```python
from build123d import *

# Parameters (mm, degrees)
F0_W      = 25.4
F0_H      = 25.4
F1_DEPTH  = 25.4
F2_W      = 20.32
F2_H      = 22.86
F3_DEPTH  = 7.62
F4_W      = 3.556
F4_H      = 20.32
F5_DEPTH  = 3.048
F6_W      = 3.556
F6_H      = 19.812
F7_DEPTH  = 3.048
F8_W      = 3.556
F8_H      = 19.812
F9_DEPTH  = 3.048
F13_DEPTH = 23.368
F12_W     = 2.54
F12_H     = 15.24
F14_DEPTH = 20.32


with BuildPart() as f1:
    # F0 (on Top) → F1 (new body)
    with BuildSketch(Plane.XY):
        Rectangle(F0_W, F0_H)
    extrude(amount=F1_DEPTH)

    # F2 (on face) → F3 (join)
    with BuildSketch(Plane(origin=(-12.7, 0, 0), x_dir=(0, -1, 0), z_dir=(-1, 0, 0))):
        with Locations((0, 11.43)):
            Rectangle(F2_W, F2_H)
    extrude(amount=F3_DEPTH)

    # F4 (on face) → F5 (cut)
    with BuildSketch(Plane.XY.offset(22.86)):
        with Locations((-16.51, 0)):
            Rectangle(F4_W, F4_H)
    extrude(amount=-F5_DEPTH, mode=Mode.SUBTRACT)

    # F6 (on face) → F7 (cut)
    with BuildSketch(Plane.XZ.offset(10.16)):
        with Locations((-16.51, 9.906)):
            Rectangle(F6_W, F6_H)
    extrude(amount=-F7_DEPTH, mode=Mode.SUBTRACT)

    # F8 (on face) → F9 (cut)
    with BuildSketch(Plane(origin=(0, 10.16, 0), x_dir=(-1, 0, 0), z_dir=(0, 1, 0))):
        with Locations((16.51, 9.906)):
            Rectangle(F8_W, F8_H)
    extrude(amount=-F9_DEPTH, mode=Mode.SUBTRACT)

    # F12 (on face) → F13 (cut)
    with BuildSketch(Plane(origin=(0, 0, 0), x_dir=(1, 0, 0), z_dir=(0, 0, -1))):
        Polygon((10.16, -7.62), (10.16, 7.62), (10.16, 10.668), (7.62, 10.668), (7.62, -10.668), (10.16, -10.668), align=None)
    extrude(amount=-F13_DEPTH, mode=Mode.SUBTRACT)

    # F12 (on face) → F14 (cut)
    with BuildSketch(Plane(origin=(0, 0, 0), x_dir=(1, 0, 0), z_dir=(0, 0, -1))):
        with Locations((11.43, 0)):
            Rectangle(F12_W, F12_H)
    extrude(amount=-F14_DEPTH, mode=Mode.SUBTRACT)


with BuildPart() as f10_1:
    # F10: copy of F1
    add(f1.part.moved(Location((-54.102, 0, 0))))


solid = f1.part
```
Model file for the job. Use its own axes, mm. A direction names the side the tool comes from. Coordinates: 2 decimals unless noted, no trailing zeros. Order: outer loops, then holes, each group sorted by start corner. A loop starts at its lowest first (then second) coordinate and runs counter-clockwise, first axis right, second up. Notation, with made-up numbers: (-19, -32.5) - (21, -32.5) arc R8 cw to (21, -24.5) - close; hole circle Ø4 at (15, -32.5). An arc over 180 degrees is marked (long way). Return JSON: item names as keys, results as strings. Group by question number.
1) Probe line 1 (X direction, y = -3.5, z = 21); line 2 (X direction, y = -7.25, z = 2); line 3 (Y direction, x = 11, z = 9.5). List the from-to ranges inside material, lowest first. Write a range as from..to.
2) Saw through at B-B, the plane z = 21.5. Write the cut outline in (x, y).
3) Mould opens along X. For faces 4 (the flat face through (-20.32, 0, 12)), 5 (the flat face through (11, 7.62, 10)), 6 (the flat face through (-17, -7.112, 10)) say: released by +X, released by -X, zero draft, split by the parting line, or undercut.
4) Tool access for faces 1 (the flat face through (9, 10.668, 12)), 2 (the flat face through (-14, -10.16, 11)), 3 (the flat face through (11, 0, 20.32)): list every direction of +Z, -Z, +X, -X, +Y, -Y with a clear straight run to the whole face (end or side of a thin tool).
5) Saw through at C-C, the plane y = -1.25. Write the cut outline in (x, z), plus the area to 3 significant figures.
6) Saw through at D-D, the plane z = 8.75. Write the cut outline in (x, y).
7) Saw through at A-A, the plane y = 9.5. Write the cut outline in (x, z), plus the area to 3 significant figures.
8) Flat gauge pins, fed straight in: P1, Ø1, axis at x = -14, z = 6.5, coming from the -Y side; P2, Ø5, axis at y = 3.5, z = 11.5, coming from the +X side; P3, Ø1.5, axis at x = -14.5, z = 17.5, coming from the +Y side. Where does each tip first touch, or does it go through?
Values found:
{
 "1": {"line 1": "x = -20.32..-18.29, -14.73..7.62, 10.16..12.7", "line 2": "x = -20.32..-18.29, -14.73..7.62", "line 3": "y = -12.7..-7.62, 7.62..12.7"},
 "2": {"outline": "(-20.32, -10.16) - (-18.29, -10.16) - (-18.29, 10.16) - (-20.32, 10.16) - close; (-14.73, -10.16) - (-12.7, -10.16) - (-12.7, -12.7) - (12.7, -12.7) - (12.7, 12.7) - (-12.7, 12.7) - (-12.7, 10.16) - (-14.73, 10.16) - close; hole (7.62, -10.67) - (10.16, -10.67) - (10.16, 10.67) - (7.62, 10.67) - close"},
 "3": {"face 4": "released by -X", "face 5": "zero draft", "face 6": "undercut"},
 "4": {"face 1": "-Z", "face 2": "+Z, -Z, -X, -Y", "face 3": "-Z, +X"},
 "5": {"outline": "(-20.32, 0) - (7.62, 0) - (7.62, 23.37) - (10.16, 23.37) - (10.16, 20.32) - (12.7, 20.32) - (12.7, 25.4) - (-12.7, 25.4) - (-12.7, 22.86) - (-14.73, 22.86) - (-14.73, 19.81) - (-18.29, 19.81) - (-18.29, 22.86) - (-20.32, 22.86) - close", "area": "698 mm²"},
 "6": {"outline": "(-20.32, -10.16) - (-18.29, -10.16) - (-18.29, -7.11) - (-14.73, -7.11) - (-14.73, -10.16) - (-12.7, -10.16) - (-12.7, -12.7) - (12.7, -12.7) - (12.7, -7.62) - (10.16, -7.62) - (10.16, -10.67) - (7.62, -10.67) - (7.62, 10.67) - (10.16, 10.67) - (10.16, 7.62) - (12.7, 7.62) - (12.7, 12.7) - (-12.7, 12.7) - (-12.7, 10.16) - (-14.73, 10.16) - (-14.73, 7.11) - (-18.29, 7.11) - (-18.29, 10.16) - (-20.32, 10.16) - close"},
 "7": {"outline": "(-20.32, 0) - (-18.29, 0) - (-18.29, 22.86) - (-20.32, 22.86) - close; (-14.73, 0) - (7.62, 0) - (7.62, 23.37) - (10.16, 23.37) - (10.16, 0) - (12.7, 0) - (12.7, 25.4) - (-12.7, 25.4) - (-12.7, 22.86) - (-14.73, 22.86) - close", "area": "679 mm²"},
 "8": {"P1": "stops at y = -10.16", "P2": "stops at x = 7.62", "P3": "stops at y = 10.16"}
}
